Study the drawing (mm; zero at the part's minimum x, y, z) and answer. Give positions to 0.01 mm unless a question says otherwise; leave off trailing zeros. Order: outer loops, then holes, each group sorted by start corner. A loop starts at its lowest first (then second) coordinate and runs counter-clockwise, first axis right, second up. Notation, with made-up numbers: (47.25, -35) - (53.25, -35) arc R28 cw to (53.25, -15) - close; hole circle Ø7 at (76.5, 88). An arc over 180 degrees is marked (long way). Write each question's results on one line, items separated by ' | '. Start each with the question number.
Q1. Find section D-D on y = 20. Give the vertices of the cut face in (x, z), and give its area (3 significant figures).
Q2. Find section B-B on y = 50. Give the vertices of the cut face in (x, z).
Q3. Find section C-C on z = 17.75. Give the vertices of the cut face in (x, y), and give its area (3 significant figures).
Q4. Flat-ended cylindrical pins translate along their axes: P1, Ø8, axis at x = 49.5, z = 6.5, coming from the +Y side; P2, Ø0.6, axis at y = 64.5, z = 10, coming from the +X side; P3, Ø0.9, axis at y = 64.5, z = 14, coming from the -X side (1 decimal). Find the tip coordinate at first contact, or state that the pin passes through.
Q5. Find the intervals of material crossed by line 1 along Y through (x, z) = (50, 15.25); line 2 along Y through (x, z) = (59.5, 18.25); line 3 along X through (y, z) = (88, 1.25) (1 decimal), in increasing order. Write a range as from..to.
Q6. Find section A-A on x = 50. Give the vertices of the cut face in (y, z).
Q7. For a pull along Y with two mould halves and no side action, classify the marked faces 1, 2 and 3 as +Y half, -Y half, draft (parallel to the pull), parting line (faces both ways), or undercut.
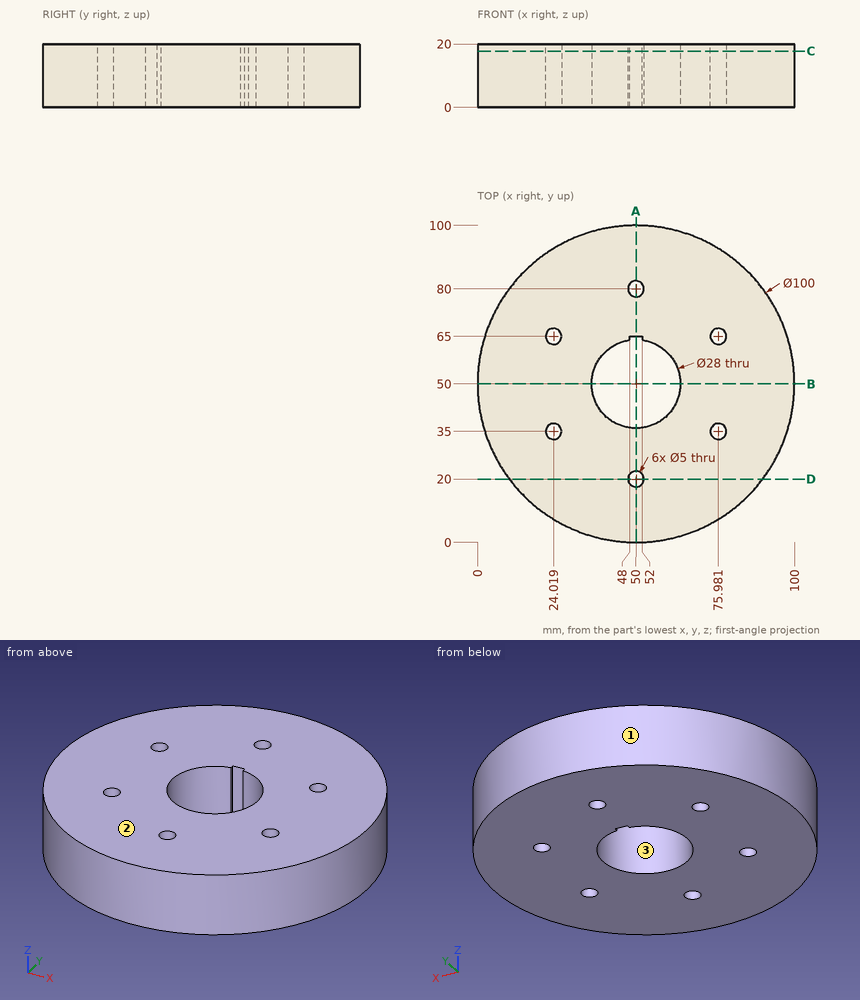
Working result:
1) outline: (10, 0) - (47.5, 0) - (47.5, 20) - (10, 20) - close; (52.5, 0) - (90, 0) - (90, 20) - (52.5, 20) - close | area: 1,500 mm²
2) outline: (0, 0) - (36, 0) - (36, 20) - (0, 20) - close; (64, 0) - (100, 0) - (100, 20) - (64, 20) - close
3) outline: circle Ø100 at (50, 50); hole circle Ø5 at (24.02, 35); hole circle Ø5 at (24.02, 65); hole circle Ø5 at (50, 20); hole circle Ø5 at (50, 80); hole (48, 63.86) arc R14 ccw (long way) to (52, 63.86) - (52, 65) - (48, 65) - close; hole circle Ø5 at (75.98, 35); hole circle Ø5 at (75.98, 65) | area: 7,120 mm²
4) P1: y = 100 | P2: x = 97.94 | P3: x = 2
5) line 1: 0..17.5, 22.5..36, 65..77.5, 82.5..100 | line 2: 0.91..39.72, 60.28..99.09 | line 3: 17.5..82.5
6) outline: (0, 0) - (17.5, 0) - (17.5, 20) - (0, 20) - close; (22.5, 0) - (36, 0) - (36, 20) - (22.5, 20) - close; (65, 0) - (77.5, 0) - (77.5, 20) - (65, 20) - close; (82.5, 0) - (100, 0) - (100, 20) - (82.5, 20) - close
7) face 1: parting line | face 2: draft | face 3: undercut
